```python
from build123d import *

# Parameters (mm, degrees)
F0_W           = 18
F0_H           = 50
F1_DEPTH       = 5
F2_R           = 1.55
F3_DEPTH       = 12.5
F5_R           = 1.55
F6_DEPTH       = 12.5
F8_D           = 3.3
F8_DEPTH       = 40
F8_CSINK_D     = 6.72
F8_CSINK_ANGLE = 90
F8_TIP         = 0.9914200214


with BuildPart() as f1:
    # F0 (on Front) → F1 (new body)
    with BuildSketch(Plane.XZ):
        with Locations((9, 25)):
            Rectangle(F0_W, F0_H)
    extrude(amount=F1_DEPTH)

    # F2 (on face) → F3 (join)
    with BuildSketch(Plane(origin=(0, 0, 0), x_dir=(1, 0, 0), z_dir=(0, 0, -1))):
        with BuildLine():
            Line((18, 0), (21.2150048465, 0))
            ThreePointArc((21.2150048465, 0), (24.1698076743, 3.5187872861), (20.1930620863, 5.8205731678))
            Line((20.1930620863, 5.8205731678), (18, 5))
            Line((18, 5), (18, 0))
        make_face()
        with Locations((21.2150048465, 3)):
            Circle(F2_R, mode=Mode.SUBTRACT)
    extrude(amount=-F3_DEPTH)

    # F5 (on offset) → F6 (join)
    with BuildSketch(Plane.XY.offset(25)):
        with BuildLine():
            Line((18, 0), (18, -5))
            Line((18, -5), (20.1930620863, -5.8205731678))
            ThreePointArc((20.1930620863, -5.8205731678), (24.1698076743, -3.5187872861), (21.2150048465, 0))
            Line((21.2150048465, 0), (18, 0))
        make_face()
        with Locations((21.2150048465, -3)):
            Circle(F5_R, mode=Mode.SUBTRACT)
    extrude(amount=F6_DEPTH)

    # F8
    with Locations(Plane.XZ.offset(5)):
        with Locations((9, 37.5), (9, 12.5)):
            CounterSinkHole(F8_D / 2, F8_CSINK_D / 2, depth=F8_DEPTH, counter_sink_angle=F8_CSINK_ANGLE)
            with Locations((0, 0, -(F8_DEPTH + F8_TIP / 2))):  # 118° drill point
                Cone(0, F8_D / 2, F8_TIP, mode=Mode.SUBTRACT)


solid = f1.part
```
Here's how the part is built. I have some questions about the finished solid (model axes, mm). A direction names the side the tool comes from. Coordinates: 2 decimals unless noted, no trailing zeros. Write each loop counter-clockwise with the first axis right and the second up, starting at its lowest first coordinate (ties: lowest second). Pieces come first, ordered by that corner, then holes. Notation, with made-up numbers: (36.25, 79) -> (61.25, 79) arc R24 cw to (61.25, 95) -> close; hole circle Ø9 at (37, 45.25). An arc over 180 degrees is marked (long way). Use a Markdown table: item, result. Add a question column.
(1) We'd pull the mould along X, two halves only. Please class faces 4 (the flat face through (19.081, -5.405, 31.162)), 5 (the flat face through (19.7, -1.6, 37.5)), 6 (the cylindrical face through (19.667, -3.068, 6.162)): +X half, -X half, draft (parallel to the pull), parting line (faces both ways), or undercut.
(2) Please list where these lines run through material, in increasing order: line 1 (Z direction, x = 20.25, y = -0.75); line 2 (Z direction, x = 9, y = -0.9); line 3 (Z direction, x = 10.5, y = -1.85).
(3) For faces 1 (the flat face through (9, -5, 25)), 2 (the flat face through (18, -2, 19)), 3 (the flat face through (18, -2, 44)), which set-ups out of +Z, -Z, +X, -X, +Y, -Y let a thin tool reach every point of the face, with its end or its side?
(4) I'm going to push flat-ended pins straight in: P1, Ø3, axis at x = 20.5, y = -3.5, coming from the +Z side; P2, Ø2, axis at x = 12.5, z = 39.5, coming from the -Y side. Where does each tip first touch, or does it pass through?
(5) If we section it at C-C, the plane x = 16.5: Write out the boundary of the cut face in (y, z).
(6) If we section it at B-B, the plane z = 24: Write out the boundary of the cut face in (x, y), and give its area (3 significant figures).
(7) If we section it at A-A, the plane x = 9: Write out the boundary of the cut face in (y, z).
Outcome:
| question | item | result |
|---|---|---|
| 1 | face 4 | -X half |
| 1 | face 5 | draft |
| 1 | face 6 | undercut |
| 2 | line 1 | z = 0 to 12.5, 25 to 37.5 |
| 2 | line 2 | z = 0 to 10.85, 14.15 to 35.85, 39.15 to 50 |
| 2 | line 3 | z = 0 to 11.81, 13.19 to 36.81, 38.19 to 50 |
| 3 | face 1 | +Z, -Z, -X, -Y |
| 3 | face 2 | +X, +Y, -Y |
| 3 | face 3 | +Z, +X, +Y, -Y |
| 4 | P1 | stops at z = 37.5 |
| 4 | P2 | stops at y = -5 |
| 5 | outline | (-5, 0) -> (0, 0) -> (0, 50) -> (-5, 50) -> close |
| 6 | outline | (0, -5) -> (18, -5) -> (18, 0) -> (0, 0) -> close |
| 6 | area | 90.0 mm^2 |
| 7 | outline | (-5, 0) -> (0, 0) -> (0, 10.85) -> (-3.29, 10.85) -> (-5, 9.14) -> close; (-5, 15.86) -> (-3.29, 14.15) -> (0, 14.15) -> (0, 35.85) -> (-3.29, 35.85) -> (-5, 34.14) -> close; (-5, 40.86) -> (-3.29, 39.15) -> (0, 39.15) -> (0, 50) -> (-5, 50) -> close |
